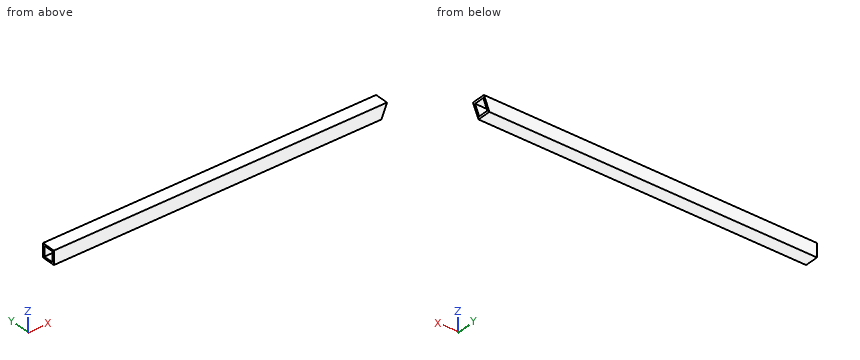
from build123d import *

# Parameters (mm, degrees)
SKETCH2_W           = 25.4
SKETCH2_H           = 25.4
SKETCH2_W_2         = 19.05
SKETCH2_H_2         = 19.05
BOSS_EXTRUDE1_DEPTH = 622.3
CUT_EXTRUDE1_REACH  = 624.948


with BuildPart() as part:
    # Sketch2 → Boss-Extrude1 (new body)
    with BuildSketch(Plane(origin=(0, 0, 0), x_dir=(0, 0, -1), z_dir=(1, 0, 0))):
        Rectangle(SKETCH2_W, SKETCH2_H)
        Rectangle(SKETCH2_W_2, SKETCH2_H_2, mode=Mode.SUBTRACT)
    extrude(amount=BOSS_EXTRUDE1_DEPTH)

    # Cut-Extrude1: up to this face of the body (flat: up to its plane)
    cut_extrude1_end = Plane(part.part.faces().sort_by_distance((311.15, -12.7, 0))[0])
    # Sketch3 → Cut-Extrude1 (cut, up to the picked face)
    with BuildSketch(Plane(origin=(0, 12.7, 0), x_dir=(1, 0, 0), z_dir=(0, 1, 0)), mode=Mode.PRIVATE) as cut_extrude1_sk1:
        Polygon((622.3, -12.7), (611.938792348, 12.7), (622.3, 12.7), align=None)
    cut_extrude1_tool1 = split(extrude(cut_extrude1_sk1.sketch, amount=-CUT_EXTRUDE1_REACH, mode=Mode.PRIVATE), bisect_by=cut_extrude1_end, keep=Keep.BOTH, mode=Mode.PRIVATE)
    add(cut_extrude1_tool1.solids().sort_by(Axis((618.846264, 12.7, -4.233333), (0, -1, 0)))[0], mode=Mode.SUBTRACT)


solid = part.part
Input: part model. Units: mm. Frame: model coordinates. Coordinates: 2 decimals unless noted, no trailing zeros. Loops run counter-clockwise (first coordinate to the right, second up) from the corner with the lowest first, then second, coordinate; pieces in that order, holes last. Notation, with made-up numbers: (-35.75, -30) - (-18.75, -30) arc R24 ccw to (-18.75, 0) - close; hole circle Ø5 at (23, 82). An arc over 180 degrees is marked (long way). Answer in a Markdown table with one row per item. Add a question column.
Item 1: Line query: line 1 along Z through (x, y) = (98.5, -1.25) (3 decimals); line 2 along X through (y, z) = (-10.25, -9.25). Output: solid intervals per line, ascending. Write a range as [from, to].
Item 2: Contact query for a flat-ended pin moving along its axis: P1, Ø6, axis at y = -8, z = 0.5, coming from the +X side. Output: stop coordinate, or through.
Item 3: Section query B-B on z = -3. Return the cut outline in (x, y) (3 decimals), then the cut area to 3 significant figures.
Item 4: Section query A-A on y = 2. Return the cut outline in (x, z) (3 decimals), then the cut area to 3 significant figures.
Item 5: Section query C-C on x = 164. Return the cut outline in (y, z) (3 decimals), then the cut area to 3 significant figures.
Recorded:
| question | item | result |
|---|---|---|
| 1 | line 1 | [-12.7, -9.525], [9.525, 12.7] |
| 1 | line 2 | [0, 613.35] |
| 2 | P1 | x = 618.38 |
| 3 | outline | (0, -12.7) - (615.896, -12.7) - (615.896, -9.525) - (0, -9.525) - close; (0, 9.525) - (615.896, 9.525) - (615.896, 12.7) - (0, 12.7) - close |
| 3 | area | 3,910 mm^2 |
| 4 | outline | (0, -12.7) - (611.939, -12.7) - (613.234, -9.525) - (0, -9.525) - close; (0, 9.525) - (621.005, 9.525) - (622.3, 12.7) - (0, 12.7) - close |
| 4 | area | 3,920 mm^2 |
| 5 | outline | (-12.7, -12.7) - (12.7, -12.7) - (12.7, 12.7) - (-12.7, 12.7) - close; hole (-9.525, -9.525) - (9.525, -9.525) - (9.525, 9.525) - (-9.525, 9.525) - close |
| 5 | area | 282 mm^2 |
